Autodesk Inventor part; units mm, degrees
ref_plane "YZ Plane" through (0, 0, 0) normal (1, 0, 0) x (0, 1, 0)
ref_plane "XZ Plane" through (0, 0, 0) normal (0, 1, 0) x (-1, 0, 0)
ref_plane "XY Plane" through (0, 0, 0) normal (0, 0, 1) x (1, 0, 0)
sketch "Sketch1" plane through (0, 0, 0) normal (0, 0, 1) x (1, 0, 0)
  circle A0 centre (0, 0) radius 20
  dimension "d0" = 40
extrude "Extrusion1" add sketch "Sketch1" along normal blind 400
sketch "Sketch2" plane through (0, 0, 0) normal (0, 1, 0) x (-1, 0, 0)
  line L0 (15, -65) -> (-15, -65)
  line L1 (-25, -40) -> (-25, 0)
  line L2 (-25, 0) -> (25, 0)
  line L3 (25, 0) -> (25, -40)
  line L4 (25, -65) -> (-25, 0) construction
  line L5 (-25, -65) -> (25, 0) construction
  line L6 (25, -40) -> (15, -65)
  line L7 (-25, -40) -> (-15, -65)
  point P0 (0, 0)
  point P1 (0, -32.5)
  dimension "d3" = 50
  dimension "d4" = 65
  dimension "d5" = 25
  dimension "d6" = 10
  dimension "d7" = 25
  dimension "d8" = 10
extrude "Extrusion2" add sketch "Sketch2" along normal mid plane 30
sketch "Sketch3" plane through (0, 15, 0) normal (0, 1, 0) x (1, 0, 0)
  point P0 (0, 0)
sketch "Sketch4" plane through (0, 0, 0) normal (0, 1, 0) x (-1, 0, 0)
  circle A0 centre (0, -40) radius 10
  line L0 (13.2288, 0) -> (-13.2288, 0)
  point P0 (0, 0)
  dimension "d11" = 20
  dimension "d12" = 40
extrude "Extrusion3" add sketch "Sketch4" along normal mid plane 60
properties part number "Parth_Pushrod"
Check sheet for the modelled part. Datum: model origin and axes. Units: mm. A direction names the side the tool comes from. Give positions to 0.01 mm unless a question says otherwise; leave off trailing zeros. Loops run counter-clockwise (first coordinate to the right, second up) from the corner with the lowest first, then second, coordinate; pieces in that order, holes last. Notation, with made-up numbers: M 65,-23 L 100,-23 A25 cw 100,-6 Z; hole C 39,67.5 d6. An arc over 180 degrees is marked long. Return JSON: item names as keys, results as strings. Group by question number.
1. Mould release check, pull along Z, two halves, no side actions. Record for faces 1 (the cylindrical face through (-4.336, 19.524, 197.2)), 2 (the cylindrical face through (2.17, 22.4, -30.24)), 3 (the flat face through (20.07, -0.21, -52.33)), 4 (the flat face through (0, 15, -25)): released by +Z, released by -Z, zero draft, split by the parting line, or undercut.
2. Go/stop test with flat-tipped pins: pin 1 (12 mm diameter, centred on y = 3.5, z = 71.5, fed in from -X); pin 2 (8 mm diameter, centred on y = 8, z = 204.5, fed in from -X); pin 3 (4 mm diameter, centred on y = 9.5, z = 215.5, fed in from -X). Record where each tip stops, or that it passes through.
3. Thickness scan on L1, parallel to X at y = -15, z = 250; L2, parallel to Y at x = 14, z = -25.5; L3, parallel to Z at x = 10.5, y = -16. Record the ranges inside material, lowest first.
4. Cross-section at D-D on y = -25. Record the boundary of the cut face in (x, z).
5. Cross-section at A-A on y = 0. Record the boundary of the cut face in (x, z), plus the area to 3 significant figures.
6. Tool access check on faces 5 (the flat face through (-22, 0, 0)), 6 (the cylindrical face through (2.17, -22.4, -49.76)), 7 (the flat face through (22, 0, 0)). Record the directions out of +Z, -Z, +X, -X, +Y, -Y that give a thin tool (end or side, any length) a straight path to the whole face; none if there is none.
7. Cross-section at C-C on z = 217.5. Record the boundary of the cut face in (x, y).
8. Cross-section at B-B on x = -2.5. Record the boundary of the cut face in (y, z).
Return value:
{
 "1": {"face 1": "zero draft", "face 2": "undercut", "face 3": "released by -Z", "face 4": "undercut"},
 "2": {"pin 1": "x = -20", "pin 2": "x = -19.6", "pin 3": "x = -18.54"},
 "3": {"L1": "-13.23 to 13.23", "L2": "-15 to 15", "L3": "0 to 400"},
 "4": {"outline": "C 0,-40 d20"},
 "5": {"outline": "M -25,-40 L -15,-65 L 15,-65 L 25,-40 L 25,0 L 20,0 L 20,400 L -20,400 L -20,0 L -25,0 Z", "area": "19,000 mm^2"},
 "6": {"face 5": "+Z, -X", "face 6": "-Y", "face 7": "+Z, +X"},
 "7": {"outline": "C 0,0 d40"},
 "8": {"outline": "M -30,-49.68 L -15,-49.68 L -15,-65 L 15,-65 L 15,-49.68 L 30,-49.68 L 30,-30.32 L 15,-30.32 L 15,0 L 19.84,0 L 19.84,400 L -19.84,400 L -19.84,0 L -15,0 L -15,-30.32 L -30,-30.32 Z"}
}
